The model under review builds one solid part; all positions refer to its coordinate system, in mm. Face numbers are marked on the shaded views. Give positions to 0.01 mm unless a question says otherwise; leave off trailing zeros. Loops run counter-clockwise (first coordinate to the right, second up) from the corner with the lowest first, then second, coordinate; pieces in that order, holes last. Notation, with made-up numbers: (-25, -27.5) - (25, -27.5) arc R22 cw to (25, 11.5) - close; hole circle Ø8 at (57.5, 65.25). An arc over 180 degrees is marked (long way). Return JSON: item names as keys, results as strings. Group by question number.
from build123d import *

# Parameters (mm, degrees)
SKETCH2_OUTSIDE_W          = 45.126
SKETCH2_OUTSIDE_H          = 45.126
CUT_EXTRUDE1_DEPTH         = 42.518512437
F_6_32_TAPPED_HOLE1_REACH  = 46.547
F_6_32_TAPPED_HOLE1_BORE_R = 1.35255
CIRPATTERN1_COUNT          = 4
F_7_8_14_TAPPED_HOLE1_D    = 20.6375


with BuildPart() as part:
    # Sketch1 → Revolve1 (revolve)
    with BuildSketch(Plane(origin=(0, 0, 0), x_dir=(0, 0, -1), z_dir=(1, 0, 0)), mode=Mode.PRIVATE) as revolve1_sk:
        with BuildLine():
            Line((-26.913863801, 11.1252), (-5.450863801, 11.1252))
            ThreePointArc((-5.450863801, 11.1252), (-4.180863801, 12.3952), (-2.910863801, 11.1252))
            Line((-2.910863801, 11.1252), (-2.910863801, 9.9695))
            Line((-2.910863801, 9.9695), (8.011136199, 9.9695))
            Line((8.011136199, 9.9695), (8.011136199, 15.875))
            Line((8.011136199, 15.875), (-26.913863801, 15.875))
            Line((-26.913863801, 15.875), (-26.913863801, 11.1252))
        make_face()
    revolve(revolve1_sk.sketch.rotate(Axis((0, 0, 0), (0, 0, 1)), 90), axis=Axis((0, 0, 0), (0, 0, 1)))

    # Sketch2 outside → Cut-Extrude1 (cut, through all)
    with BuildSketch(Plane.XY.offset(26.913863801)):
        Rectangle(SKETCH2_OUTSIDE_W, SKETCH2_OUTSIDE_H)
        Polygon((0, -21.328108288), (-21.328108288, 0), (0, 21.328108288), (21.328108288, 0), align=None, mode=Mode.SUBTRACT)
    extrude(amount=-CUT_EXTRUDE1_DEPTH, mode=Mode.SUBTRACT)

    # 6-32 Tapped Hole1 bore → 6-32 Tapped Hole1 (cut, up to next)
    with BuildSketch(Plane(origin=(15.875, 0, 0), x_dir=(0, 0, -1), z_dir=(1, 0, 0)), mode=Mode.PRIVATE) as f_6_32_tapped_hole1_sk1:
        with Locations((-20.563863801, 0)):
            Circle(F_6_32_TAPPED_HOLE1_BORE_R)
    f_6_32_tapped_hole1_tool1 = extrude(f_6_32_tapped_hole1_sk1.sketch, amount=-F_6_32_TAPPED_HOLE1_REACH, mode=Mode.PRIVATE) & part.part
    # 6-32 Tapped Hole1 bore → 6-32 Tapped Hole1 (cut, up to next)
    with BuildSketch(Plane(origin=(15.875, 0, 0), x_dir=(0, 0, -1), z_dir=(1, 0, 0)), mode=Mode.PRIVATE) as f_6_32_tapped_hole1_sk2:
        with Locations((-14.213863801, 0)):
            Circle(F_6_32_TAPPED_HOLE1_BORE_R)
    f_6_32_tapped_hole1_tool2 = extrude(f_6_32_tapped_hole1_sk2.sketch, amount=-F_6_32_TAPPED_HOLE1_REACH, mode=Mode.PRIVATE) & part.part
    f_6_32_tapped_hole1_1 = f_6_32_tapped_hole1_tool1.solids().sort_by_distance((15.875, 0, 20.563864))[0]
    add(f_6_32_tapped_hole1_1, mode=Mode.SUBTRACT)
    f_6_32_tapped_hole1_2 = f_6_32_tapped_hole1_tool2.solids().sort_by_distance((15.875, 0, 14.213864))[0]
    add(f_6_32_tapped_hole1_2, mode=Mode.SUBTRACT)
    f_6_32_tapped_hole1 = f_6_32_tapped_hole1_1 + f_6_32_tapped_hole1_2  # 6-32 Tapped Hole1 as one shape, for the pattern or mirror that repeats it

    # CirPattern1: 6-32 Tapped Hole1 ×4 about axis
    cirpattern1_axis = Axis((0, 0, 0), (0, 0, -1))
    for i in range(1, CIRPATTERN1_COUNT):
        add(f_6_32_tapped_hole1.rotate(cirpattern1_axis, i * 360 / CIRPATTERN1_COUNT), mode=Mode.SUBTRACT)

    # 7_8-14 Tapped Hole1 (through all)
    with Locations(Plane(origin=(0, 0, -8.011136199), x_dir=(-1, 0, 0), z_dir=(0, 0, -1))):
        with Locations((0, 0)):
            Hole(F_7_8_14_TAPPED_HOLE1_D / 2)


solid = part.part
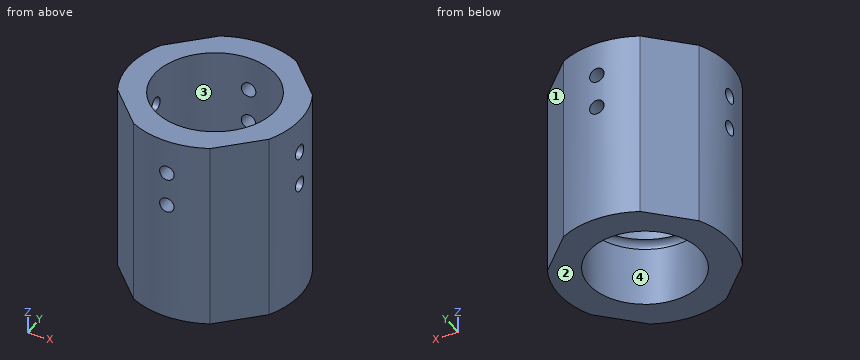
Item 1: Take a section at B-B (z = 8). State the section outline as (x, y) points (3 decimals), then the cut area to 3 significant figures.
Item 2: Mouldability with a two-part tool opening along Y and no side actions: class the marked faces 1, 2, 3 and 4 as +Y half, -Y half, draft (parallel to the pull), parting line (faces both ways), or undercut.
Item 3: For L1, parallel to Z at x = 0, y = 13.85; L2, parallel to Y at x = 0, z = -3 (3 decimals); L3, parallel to X at y = 0, z = 16 (3 decimals), list the stretches that pass through material, from the lowest coordinate up. Write a range as from..to.
Item 4: Take a section at A-A (x = 0). State how many separate pieces and enclosed holes the cut face has, then the cut area to 3 significant figures.
Item 5: For P1, Ø11, axis at x = -2, y = -3, coming from the +Z side; P2, Ø12, axis at x = -9, z = -3.5, coming from the +Y side; P3, Ø6, axis at x = -12, z = 2.5, coming from the -Y side; P4, Ø1.5, axis at x = 7.5, z = -2, coming from the +Y side, all flat-tipped, find the tip position at first contact; note any pin that passes through.
Check sheet entries:
{
 "1": {"outline": "(-14.169, -7.159) - (-7.159, -14.169) arc R15.875 ccw to (7.159, -14.169) - (14.169, -7.159) arc R15.875 ccw to (14.169, 7.159) - (7.159, 14.169) arc R15.875 ccw to (-7.159, 14.169) - (-14.169, 7.159) arc R15.875 ccw to start; hole circle Ø22.25 at (0, 0)", "area": "382 mm^2"},
 "2": {"face 1": "+Y half", "face 2": "draft", "face 3": "undercut", "face 4": "undercut"},
 "3": {"L1": "z = -8.01..12.86, 15.57..19.21, 21.92..26.91", "L2": "y = -15.875..-10.319, 10.319..15.875", "L3": "x = -15.875..-11.125, 11.125..15.875"},
 "4": {"separate pieces": "6", "enclosed holes": "0", "area": "293 mm^2"},
 "5": {"P1": "passes through", "P2": "stops at y = 15.59", "P3": "stops at y = -12.33", "P4": "stops at y = 14.37"}
}
